Geometry check sheet. Reference: the model listing, model coordinates, mm. Give positions to 0.01 mm unless a question says otherwise; leave off trailing zeros. Write each loop counter-clockwise with the first axis right and the second up, starting at its lowest first coordinate (ties: lowest second). Pieces come first, ordered by that corner, then holes. Notation, with made-up numbers: (59, 8.5) - (96, 8.5) arc R36 cw to (96, 43.5) - close; hole circle Ø3 at (7, 9). An arc over 180 degrees is marked (long way). Use a Markdown table: item, result.
```python
from build123d import *

# Parameters (mm, degrees)
F1_DEPTH       = 25.4
F3_D           = 6.35
F3_CSINK_D     = 12.7
F3_CSINK_ANGLE = 90
F4_R           = 1.27
F5_SIZE        = 5.08


with BuildPart() as f1:
    # F0 (on Top) → F1 (new body)
    with BuildSketch(Plane.XY):
        with BuildLine():
            ThreePointArc((-27.760715, 26.09507), (-14.034364, -35.420991), (38.1, 0))
            ThreePointArc((38.1, 0), (14.034364, 35.420991), (-27.760715, 26.09507))
        make_face()
    extrude(amount=F1_DEPTH)

    # F3 (through all)
    with Locations(Plane.XY.offset(25.4)):
        with Locations((-12.7, 0), (0, 12.7), (12.7, 0)):
            CounterSinkHole(F3_D / 2, F3_CSINK_D / 2, counter_sink_angle=F3_CSINK_ANGLE)

    # F4
    f4_edges = [f1.edges().sort_by_distance(p)[0] for p in [
        (-38.1, 0, 25.4),
    ]]
    fillet(f4_edges, radius=F4_R)

    # F5
    f5_edges = [f1.edges().sort_by_distance(p)[0] for p in [
        (-38.1, 0, 0),
    ]]
    chamfer(f5_edges, length=F5_SIZE)


solid = f1.part
```
1) Material ranges on L1, parallel to X at y = -0.5, z = 10.25; L2, parallel to X at y = 12.7, z = 15 (3 decimals), recorded low to high. Write a range as from..to.
Working result:
| item | result |
|---|---|
| L1 | x = -38.1..-15.84, -9.56..9.56, 15.84..38.1 |
| L2 | x = -35.921..-3.175, 3.175..35.921 |
2) Depth check by flat-ended pin: P1, Ø4, axis at y = -21.5, z = 5.5, coming from the -X side; P2, Ø4, axis at y = 9, z = 7.5, coming from the -X side; P3, Ø6, axis at y = -19, z = 19, coming from the -X side. Enter the tip coordinate at first touch or a pass-through.
Working result:
| item | result |
|---|---|
| P1 | stops at x = -32.73 |
| P2 | stops at x = -37.45 |
| P3 | stops at x = -34.58 |
3) Section check B-B on z = 3.5. Record the boundary of the cut face in (x, y) (3 decimals).
Working result:
| item | result |
|---|---|
| outline | circle Ø73.04 at (0, 0); hole circle Ø6.35 at (-12.7, 0); hole circle Ø6.35 at (0, 12.7); hole circle Ø6.35 at (12.7, 0) |
4) Mould release check, pull along Y, two halves, no side actions. Record for faces 1 (the flat face through (0, 0, 0)), 2 (the conical face through (11.16, -2.95, 22.38)): pulls with the +Y half, pulls with the -Y half, needs draft (parallel to the pull), parting line crosses it, or undercut.
Working result:
| item | result |
|---|---|
| face 1 | needs draft |
| face 2 | undercut |
5) Section check A-A on z = 9.5. Record the boundary of the cut face in (x, y) (3 decimals).
Working result:
| item | result |
|---|---|
| outline | circle Ø76.2 at (0, 0); hole circle Ø6.35 at (-12.7, 0); hole circle Ø6.35 at (0, 12.7); hole circle Ø6.35 at (12.7, 0) |
